Build history of the part. All positions in model axes, mm. Give positions to 0.01 mm unless a question says otherwise; leave off trailing zeros. Order: outer loops, then holes, each group sorted by start corner. A loop starts at its lowest first (then second) coordinate and runs counter-clockwise, first axis right, second up. Notation, with made-up numbers: (35, 80) - (64, 80) arc R7 ccw to (64, 86) - close; hole circle Ø5 at (57.5, -6). An arc over 180 degrees is marked (long way). Use a Markdown table: item, result.
from build123d import *

# Parameters (mm, degrees)
SKETCH1_R           = 4
SKETCH1_R_2         = 5
BOSS_EXTRUDE1_DEPTH = 3


with BuildPart() as part:
    # Sketch1 → Boss-Extrude1 (new body)
    with BuildSketch(Plane.XY):
        with BuildLine():
            Line((-80.425564374, 96.680246319), (-69.786632227, 96.680246319))
            ThreePointArc((-69.786632227, 96.680246319), (-67.144628902, 97.774599928), (-66.050275293, 100.416603253))
            Line((-66.050275293, 100.416603253), (-66.050275293, 142.972331842))
            ThreePointArc((-66.050275293, 142.972331842), (-67.144628902, 145.614335167), (-69.786632227, 146.708688776))
            Line((-69.786632227, 146.708688776), (-80.425564374, 146.708688776))
            ThreePointArc((-80.425564374, 146.708688776), (-83.067567699, 145.614335167), (-84.161921308, 142.972331842))
            Line((-84.161921308, 142.972331842), (-84.161921308, 100.416603253))
            ThreePointArc((-84.161921308, 100.416603253), (-83.067567699, 97.774599928), (-80.425564374, 96.680246319))
        make_face()
        with Locations((-75.106098301, 104.343716036)):
            Circle(SKETCH1_R, mode=Mode.SUBTRACT)
        with Locations((-75.106098301, 116.730443274)):
            Circle(SKETCH1_R, mode=Mode.SUBTRACT)
        with Locations((-75.106098301, 135.57981081)):
            Circle(SKETCH1_R_2, mode=Mode.SUBTRACT)
    extrude(amount=BOSS_EXTRUDE1_DEPTH)


solid = part.part
1) Wall check: line 1 (Y direction, x = -74, z = 1.2); line 2 (Y direction, x = -73.75, z = 2.1); line 3 (X direction, y = 105.5, z = 0.95). Give the ranges that are in metal, low to high. Write a range as from..to.
Computed:
| item | result |
|---|---|
| line 1 | y = 96.68..100.5, 108.19..112.89, 120.57..130.7, 140.46..146.71 |
| line 2 | y = 96.68..100.58, 108.11..112.97, 120.49..130.77, 140.39..146.71 |
| line 3 | x = -84.16..-78.94, -71.28..-66.05 |
2) Slice it at A-A (x = -75.5). Write the cut outline in (y, z).
Computed:
| item | result |
|---|---|
| outline | (96.68, 0) - (100.36, 0) - (100.36, 3) - (96.68, 3) - close; (108.32, 0) - (112.75, 0) - (112.75, 3) - (108.32, 3) - close; (120.71, 0) - (130.6, 0) - (130.6, 3) - (120.71, 3) - close; (140.56, 0) - (146.71, 0) - (146.71, 3) - (140.56, 3) - close |
3) Slice it at D-D (x = -73.25). Write the cut outline in (y, z).
Computed:
| item | result |
|---|---|
| outline | (96.68, 0) - (100.8, 0) - (100.8, 3) - (96.68, 3) - close; (107.89, 0) - (113.19, 0) - (113.19, 3) - (107.89, 3) - close; (120.27, 0) - (130.94, 0) - (130.94, 3) - (120.27, 3) - close; (140.22, 0) - (146.71, 0) - (146.71, 3) - (140.22, 3) - close |
4) Slice it at C-C (z = 0.6). Write the cut outline in (x, y), and give its area (3 significant figures).
Computed:
| item | result |
|---|---|
| outline | (-84.16, 100.42) arc R3.74 ccw to (-80.43, 96.68) - (-69.79, 96.68) arc R3.74 ccw to (-66.05, 100.42) - (-66.05, 142.97) arc R3.74 ccw to (-69.79, 146.71) - (-80.43, 146.71) arc R3.74 ccw to (-84.16, 142.97) - close; hole circle Ø10 at (-75.11, 135.58); hole circle Ø8 at (-75.11, 104.34); hole circle Ø8 at (-75.11, 116.73) |
| area | 715 mm² |
5) Two-plate mould, pull along X, no slides. Class faces 1 (the flat face through (-66.05, 121, 1)), 2 (the cylindrical face through (-83.096, 97.804, 1.479)), 3 (the cylindrical face through (-75.757, 140.537, 1.479)): +X half, -X half, draft (parallel to the pull), parting line (faces both ways), or undercut.
Computed:
| item | result |
|---|---|
| face 1 | +X half |
| face 2 | -X half |
| face 3 | undercut |
6) Slice it at B-B (y = 135). Write the cut outline in (x, z), and give its area (3 significant figures).
Computed:
| item | result |
|---|---|
| outline | (-84.16, 0) - (-80.07, 0) - (-80.07, 3) - (-84.16, 3) - close; (-70.14, 0) - (-66.05, 0) - (-66.05, 3) - (-70.14, 3) - close |
| area | 24.5 mm² |
